Source: CAD feature listing. Evaluate the final solid. Frame: model axes, mm. Face numbers are marked on the shaded views. A direction names the side the tool comes from. Round coordinates to 2 decimals unless told otherwise and drop trailing zeros. Write each loop counter-clockwise with the first axis right and the second up, starting at its lowest first coordinate (ties: lowest second). Pieces come first, ordered by that corner, then holes. Notation, with made-up numbers: (41.25, -34.75) -> (50.25, -34.75) arc R8 cw to (50.25, -25.75) -> close; hole circle Ø1 at (34, -29.75). An arc over 180 degrees is marked (long way). Put each result on its own line as item: value.
Autodesk Inventor part; units mm, degrees
ref_plane "YZ Plane" through (0, 0, 0) normal (1, 0, 0) x (0, 1, 0)
ref_plane "XZ Plane" through (0, 0, 0) normal (0, 1, 0) x (-1, 0, 0)
ref_plane "XY Plane" through (0, 0, 0) normal (0, 0, 1) x (1, 0, 0)
sketch "Sketch1" plane through (0, 0, 0) normal (0, 0, 1) x (1, 0, 0)
  line L0 (88, 5) -> (88, 7)
  line L1 (0, 7) -> (0, 5)
  line L2 (0, 0) -> (0, 32) construction
  line L3 (0, 32) -> (28, 32) construction
  line L4 (28, 32) -> (60, 32) construction
  line L5 (60, 32) -> (88, 32) construction
  line L6 (88, 32) -> (88, 0) construction
  line L7 (60, 63.7192) -> (60, -36.6397) construction
  line L8 (28, 67.21) -> (28, -43.6212) construction
  line L9 (44, 32) -> (44, 16) construction
  line L10 (27.7, 5) -> (27.7, 16)
  arc A0 (60.3, 16) -> (27.7, 16) centre (44, 16) ccw
  line L11 (60.3, 16) -> (60.3, 5)
  arc A1 (65.223, 20.9825) -> (22.777, 20.9825) centre (44, 16) ccw
  line L12 (22.2, 7) -> (13.2, 7)
  line L13 (22.2, 0) -> (22.2, 5)
  line L14 (22.2, 5) -> (0, 5)
  line L15 (0, 5) -> (0, 12)
  line L16 (88, 12) -> (88, 5)
  line L17 (22.2, 7) -> (13.2, 7)
  arc A2 (14, 12) -> (22.777, 20.9825) centre (8.2155, 26.4316) ccw
  arc A3 (65.223, 20.9825) -> (74, 12) centre (79.7845, 26.4316) ccw
  line L18 (60.3, 7) -> (60, 7)
  line L19 (28, 7) -> (27.7, 7)
  line L20 (22.2, 5) -> (28, 5)
  line L21 (60, 5) -> (88, 5)
  line L22 (27.7, 0) -> (28, 0)
  line L23 (60, 0) -> (60.3, 0)
  line L24 (0, 12) -> (14, 12)
  line L25 (27.7, 12) -> (28, 12)
  line L26 (22.2, 0) -> (22.2, 7)
  line L27 (60, 12) -> (60.3, 12)
  line L28 (74, 12) -> (88, 12)
  dimension "d0" = 88
  dimension "d1" = 7
  dimension "d2" = 32
  dimension "d3" = 28
  dimension "d4" = 32
  dimension "d5" = 28
  dimension "d6" = 16
  dimension "d8" = 5.5
  dimension "d9" = 9
  dimension "d10" = 5
  dimension "d11" = 7
  dimension "d12" = 9
extrude "Extrusion1" add sketch "Sketch1" along normal blind 28
sketch "Sketch2" plane through (0, 12, 0) normal (0, 1, 0) x (1, 0, 0)
  line L0 (14, 0) -> (0, 0)
  line L1 (14, 0) -> (14, -28)
  line L2 (0, 0) -> (14, -28) construction
  line L3 (14, 0) -> (0, -28) construction
  line L4 (7, 0) -> (7, -7) construction
  circle A0 centre (7, -7) radius 2.743
  dimension "d15" = 7
  dimension "d16" = 5.486
extrude "Extrusion2" cut sketch "Sketch2" against normal blind 28
ref_plane "Work Plane1" through (0, 0, 14) normal (0, 0, 1) x (1, 0, 0)
ref_plane "Work Plane2" through (44, 5, 0) normal (-1, 0, 0) x (0, 0, 1)
mirror "Mirror1" about plane through (0, 0, 14) normal (0, 0, 1) of "Extrusion2"
mirror "Mirror2" about plane through (44, 5, 0) normal (-1, 0, 0) of "Extrusion2", "Mirror1"
sketch "Sketch3" plane through (0, 12, 0) normal (0, 1, 0) x (1, 0, 0)
  circle A0 centre (7, -21) radius 2.743
  circle A1 centre (7, -7) radius 2.743
  line L0 (14, 0) -> (0, 0)
  line L1 (0, 0) -> (0, -28)
  line L2 (14, -28) -> (0, -28)
  line L3 (14, 0) -> (14, -28)
  circle A2 centre (7, -7) radius 3.143
  circle A3 centre (7, -7) radius 2.743
  dimension "d19" = 0.4
extrude "Extrusion3" cut sketch "Sketch3" against normal blind 10 contours A2
mirror "Mirror3" about plane through (0, 0, 14) normal (0, 0, 1) of "Extrusion3"
mirror "Mirror4" about plane through (44, 5, 0) normal (-1, 0, 0) of "Extrusion3", "Mirror3"
properties part number "Motor Mount"
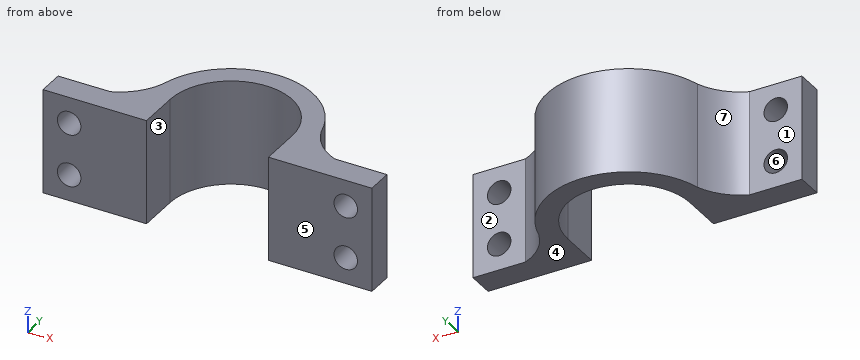
Q1. Pin query (flat end, axial travel): pin 1 (12 mm diameter, centred on y = 25.5, z = 10, fed in from -X); pin 2 (15.5 mm diameter, centred on x = 5.5, z = 19.5, fed in from +Y); pin 3 (12 mm diameter, centred on x = 62.5, z = 22, fed in from +Y). Return the tip coordinate at first contact, or that it passes through.
Ans:
pin 1: stops at x = 22.13
pin 2: stops at y = 12
pin 3: stops at y = 33.86
Q2. Material intervals for line 1 (Z direction, x = 7, y = 10); line 2 (X direction, y = 10.25, z = 7); line 3 (X direction, y = 9, z = 15), sorted ascending. Write a range as [from, to].
Ans:
line 1: z = [0, 3.86], [10.14, 17.86], [24.14, 28]
line 2: x = [0, 3.86], [10.14, 27.7], [60.3, 77.86], [84.14, 88]
line 3: x = [0, 27.7], [60.3, 88]
Q3. Reachability of the marked faces 1, 2, 3 and 4 from +Z, -Z, +X, -X, +Y, -Y: full face, straight path, thin tool, end or side. Return the list, or none.
Ans:
face 1: +Z, -Z, -X, +Y
face 2: +Z, -Z, +X, +Y
face 3: +Z, -Z, -Y
face 4: -Z, +X, -X, +Y, -Y
Q4. Draft query along X for the marked faces 5, 6 and 7. Return one class per face: +X half, -X half, draft (parallel to the pull), parting line (faces both ways), or undercut.
Ans:
face 5: draft
face 6: undercut
face 7: -X half
Q5. Cut plane A-A on z = 7. Output: boundary loops of the cut face in (x, y), and give its area (3 significant figures).
Ans:
outline: (0, 5) -> (3.86, 5) -> (3.86, 12) -> (0, 12) -> close; (10.14, 5) -> (27.7, 5) -> (27.7, 16) arc R16.3 cw to (60.3, 16) -> (60.3, 5) -> (77.86, 5) -> (77.86, 12) -> (74, 12) arc R15.55 cw to (65.22, 20.98) arc R21.8 ccw to (22.78, 20.98) arc R15.55 cw to (14, 12) -> (10.14, 12) -> close; (84.14, 5) -> (88, 5) -> (88, 12) -> (84.14, 12) -> close
area: 721 mm^2
Q6. Cut plane D-D on y = 17. Output: boundary loops of the cut face in (x, z).
Ans:
outline: (20.58, 0) -> (27.73, 0) -> (27.73, 28) -> (20.58, 28) -> close; (60.27, 0) -> (67.42, 0) -> (67.42, 28) -> (60.27, 28) -> close
Q7. Cut plane B-B on y = 10. Output: boundary loops of the cut face in (x, z).
Ans:
outline: (0, 0) -> (27.7, 0) -> (27.7, 28) -> (0, 28) -> close; (60.3, 0) -> (88, 0) -> (88, 28) -> (60.3, 28) -> close; hole circle Ø6.29 at (7, 7); hole circle Ø6.29 at (7, 21); hole circle Ø6.29 at (81, 7); hole circle Ø6.29 at (81, 21)
Q8. Cut plane C-C on x = 7. Output: boundary loops of the cut face in (y, z).
Ans:
outline: (5, 0) -> (12, 0) -> (12, 3.86) -> (5, 3.86) -> close; (5, 10.14) -> (12, 10.14) -> (12, 17.86) -> (5, 17.86) -> close; (5, 24.14) -> (12, 24.14) -> (12, 28) -> (5, 28) -> close
